Input: part model. Units: mm. Frame: model coordinates. A direction names the side the tool comes from. Coordinates: 2 decimals unless noted, no trailing zeros. Write each loop counter-clockwise with the first axis right and the second up, starting at its lowest first coordinate (ties: lowest second). Pieces come first, ordered by that corner, then holes. Notation, with made-up numbers: M 48,79.5 L 56,79.5 A4 cw 56,84.5 Z; hole C 1,-18.75 d3. An arc over 180 degrees is marked long. Write each question's results on one line, items separated by ' | '. Start each with the question number.
1. Pull-direction query (Y, two-part tool) for faces 4 (the flat face through (-22, 7, -12.85)), 5 (the flat face through (-17.514, 5, -10)), 6 (the flat face through (22.38, 2.52, 11.405)); classes: +Y half, -Y half, draft (parallel to the pull), parting line (faces both ways), or undercut.
2. First-contact query: pin 1 (2.5 mm diameter, centred on x = -10, z = 7.5, fed in from +Y); pin 2 (1 mm diameter, centred on y = 5.5, z = 9, fed in from +X). Flat tips, straight axial feed; report the tip coordinate or a pass-through.
3. Section query D-D, the plane x = 10. Output: boundary loops of the cut face in (y, z), and give its area (3 significant figures).
4. Set-up query: faces 1 (the cylindrical face through (19.39, 3.536, 9.239)), 2 (the flat face through (22.38, 2.54, 8.56)), 3 (the cylindrical face through (16.283, 5.07, -1.959)). Return all of +Z, -Z, +X, -X, +Y, -Y with unobstructed straight access to the full face (end or side cutting, diameter ignored); none if empty.
5. Section query C-C, the plane y = 2.75. Count the separate pieces of the cut face and the enclosed holes in it, and give its area (3 significant figures).
6. Section query A-A, the plane z = -1.2. Output: boundary loops of the cut face in (x, y), and give its area (3 significant figures).
7. Section query B-B, the plane x = 19.7. Output: boundary loops of the cut face in (y, z), and give its area (3 significant figures).
8. Ray query, probe 1 along X at (y, z) = (7.75, -12.75); probe 2 along Z at (x, y) = (-26.85, 5); probe 3 along X at (y, z) = (3.75, -1.2). Return the intervals inside material, ascending.
```python
from build123d import *

# Parameters (mm, degrees)
SKETCH1_W           = 59.0272
SKETCH1_H           = 30
BOSS_EXTRUDE1_DEPTH = 10
SKETCH2_R           = 2.1
CUT_EXTRUDE1_DEPTH  = 35.58399319
SKETCH3_R           = 1.65
CUT_EXTRUDE2_DEPTH  = 12
CUT_EXTRUDE3_START  = -12
SKETCH4_R           = 1.65
CUT_EXTRUDE3_DEPTH  = 12
CUT_EXTRUDE4_DEPTH  = 2.3
CUT_EXTRUDE5_DEPTH  = 2.3
SKETCH7_R           = 3.5
CUT_EXTRUDE6_DEPTH  = 35.58399319


with BuildPart() as part:
    # Sketch1 → Boss-Extrude1 (new body)
    with BuildSketch(Plane(origin=(0, 0, 0), x_dir=(1, 0, 0), z_dir=(0, 1, 0))):
        Rectangle(SKETCH1_W, SKETCH1_H)
    extrude(amount=BOSS_EXTRUDE1_DEPTH)

    # Sketch2 → Cut-Extrude1 (cut, through all)
    with BuildSketch(Plane(origin=(0, 10, 0), x_dir=(1, 0, 0), z_dir=(0, 1, 0))):
        with Locations(Location((-10, -7.5, 0), (0, 0, 270))):
            Circle(SKETCH2_R)
        with Locations(Location((10, -7.5, 0), (0, 0, 270))):
            Circle(SKETCH2_R)
    extrude(amount=-CUT_EXTRUDE1_DEPTH, mode=Mode.SUBTRACT)

    # Sketch3 → Cut-Extrude2 (cut)
    with BuildSketch(Plane(origin=(29.5136, 0, 0), x_dir=(0, 0, -1), z_dir=(1, 0, 0))):
        with Locations((-10, 5)):
            Circle(SKETCH3_R)
        with Locations((10, 5)):
            Circle(SKETCH3_R)
    extrude(amount=-CUT_EXTRUDE2_DEPTH, mode=Mode.SUBTRACT)

    # Sketch4 → Cut-Extrude3 (cut)
    with BuildSketch(Plane.ZY.offset(29.5136).offset(CUT_EXTRUDE3_START)):
        with Locations(Location((-10, 5, 0), (0, 0, 180))):
            Circle(SKETCH4_R)
        with Locations(Location((10, 5, 0), (0, 0, 180))):
            Circle(SKETCH4_R)
    extrude(amount=CUT_EXTRUDE3_DEPTH, mode=Mode.SUBTRACT)

    # Sketch5 → Cut-Extrude4 (cut)
    with BuildSketch(Plane(origin=(23.5136, 0, 0), x_dir=(0, 0, -1), z_dir=(1, 0, 0))):
        Polygon((-12.85, 6.645448267), (-12.85, 10), (-7.15, 10), (-7.15, 6.645448267), (-7.15, 3.354551733), (-10, 1.709103466), (-12.85, 3.354551733), align=None)
        Polygon((7.15, 6.645448267), (7.15, 3.354551733), (10, 1.709103466), (12.85, 3.354551733), (12.85, 6.645448267), (12.85, 10), (7.15, 10), align=None)
    extrude(amount=-CUT_EXTRUDE4_DEPTH, mode=Mode.SUBTRACT)

    # Sketch6 → Cut-Extrude5 (cut)
    with BuildSketch(Plane.ZY.offset(23.5136)):
        Polygon((-12.85, 6.645448267), (-12.85, 10), (-7.15, 10), (-7.15, 6.645448267), (-7.15, 3.354551733), (-10, 1.709103466), (-12.85, 3.354551733), align=None)
        Polygon((7.15, 6.645448267), (7.15, 3.354551733), (10, 1.709103466), (12.85, 3.354551733), (12.85, 6.645448267), (12.85, 10), (7.15, 10), align=None)
    extrude(amount=-CUT_EXTRUDE5_DEPTH, mode=Mode.SUBTRACT)

    # Sketch7 → Cut-Extrude6 (cut, through all)
    with BuildSketch(Plane(origin=(0, 10, 0), x_dir=(1, 0, 0), z_dir=(0, 1, 0))):
        with Locations(Location((19.7, 1.2, 0), (0, 0, 270))):
            Circle(SKETCH7_R)
        with Locations(Location((-5.7, 1.2, 0), (0, 0, 270))):
            Circle(SKETCH7_R)
    extrude(amount=-CUT_EXTRUDE6_DEPTH, mode=Mode.SUBTRACT)


solid = part.part
```
Answer:
1) face 4: draft | face 5: undercut | face 6: +Y half
2) pin 1: through | pin 2: x = 17.51
3) outline: M 0,-15 L 10,-15 L 10,5.4 L 0,5.4 Z; M 0,9.6 L 10,9.6 L 10,15 L 0,15 Z | area: 258 mm^2
4) face 1: +X | face 2: +Y | face 3: +Y, -Y
5) separate pieces: 1 | enclosed holes: 8 | area: 1,630 mm^2
6) outline: M -29.51,0 L -9.2,0 L -9.2,10 L -29.51,10 Z; M -2.2,0 L 16.2,0 L 16.2,10 L -2.2,10 Z; M 23.2,0 L 29.51,0 L 29.51,10 L 23.2,10 Z | area: 450 mm^2
7) outline: M 0,-15 L 10,-15 L 10,-4.7 L 0,-4.7 Z; M 0,2.3 L 10,2.3 L 10,15 L 0,15 Z; hole C 5,-10 d3.3; hole C 5,10 d3.3 | area: 213 mm^2
8) probe 1: -29.51 to -23.51, -21.21 to 21.21, 23.51 to 29.51 | probe 2: -15 to -11.65, -8.35 to 8.35, 11.65 to 15 | probe 3: -29.51 to -9.2, -2.2 to 16.2, 23.2 to 29.51
